```python
from build123d import *

# Parameters (mm, degrees)
SKETCH1_R           = 10
SKETCH1_R_2         = 1.5
SKETCH1_R_3         = 4.5
BOSS_EXTRUDE1_DEPTH = 2
SKETCH1_2_R         = 4.5
BOSS_EXTRUDE2_DEPTH = 4.5
SKETCH2_R           = 1.5
CUT_EXTRUDE1_DEPTH  = 4.5
SKETCH3_R           = 2.75
CUT_EXTRUDE2_DEPTH  = 3.5
CUT_EXTRUDE3_DEPTH  = 3.5
CIRPATTERN1_COUNT   = 25


with BuildPart() as part:
    # Sketch1 → Boss-Extrude1 (new body)
    with BuildSketch(Plane.XY):
        Circle(SKETCH1_R)
        with Locations((0, 7)):
            Circle(SKETCH1_R_2, mode=Mode.SUBTRACT)
        with Locations((7, 0)):
            Circle(SKETCH1_R_2, mode=Mode.SUBTRACT)
        with Locations((0, -7)):
            Circle(SKETCH1_R_2, mode=Mode.SUBTRACT)
        with Locations((-7, 0)):
            Circle(SKETCH1_R_2, mode=Mode.SUBTRACT)
        Circle(SKETCH1_R_3, mode=Mode.SUBTRACT)
    extrude(amount=BOSS_EXTRUDE1_DEPTH)

    # Sketch1_2 → Boss-Extrude2 (add)
    with BuildSketch(Plane.XY):
        Circle(SKETCH1_2_R)
    extrude(amount=BOSS_EXTRUDE2_DEPTH)

    # Sketch2 → Cut-Extrude1 (cut)
    with BuildSketch(Plane(origin=(0, 0, 0), x_dir=(-1, 0, 0), z_dir=(0, 0, -1))):
        Circle(SKETCH2_R)
    extrude(amount=-CUT_EXTRUDE1_DEPTH, mode=Mode.SUBTRACT)

    # Sketch3 → Cut-Extrude2 (cut)
    with BuildSketch(Plane.XY.offset(4.5)):
        Circle(SKETCH3_R)
    extrude(amount=-CUT_EXTRUDE2_DEPTH, mode=Mode.SUBTRACT)

    # Sketch4 → Cut-Extrude3 (cut)
    with BuildSketch(Plane.XY.offset(4.5)):
        with BuildLine():
            Line((-2.976344104, 0.375999701), (-2.728315429, 0.344666392))
            ThreePointArc((-2.728315429, 0.344666392), (-2.70218519, 0.510583192), (-2.665974712, 0.674595311))
            Line((-2.665974712, 0.674595311), (-2.976344104, 0.375999701))
        make_face()
        with BuildLine():
            Line((-2.976344104, 0.375999701), (-2.75, 0))
            ThreePointArc((-2.75, 0), (-2.744573503, 0.172673929), (-2.728315429, 0.344666392))
            Line((-2.728315429, 0.344666392), (-2.976344104, 0.375999701))
        make_face()
    cut_extrude3 = extrude(amount=-CUT_EXTRUDE3_DEPTH, mode=Mode.SUBTRACT)

    # CirPattern1: Cut-Extrude3 ×25 about axis
    cirpattern1_axis = Axis((0, 0, 0), (0, 0, 1))
    for i in range(1, CIRPATTERN1_COUNT):
        add(cut_extrude3.rotate(cirpattern1_axis, i * 360 / CIRPATTERN1_COUNT), mode=Mode.SUBTRACT)


solid = part.part
```
The listing builds one solid part. Answer for the finished solid, in the listing's coordinates (mm). A direction names the side the tool comes from. Round coordinates to 2 decimals unless told otherwise and drop trailing zeros. Write each loop counter-clockwise with the first axis right and the second up, starting at its lowest first coordinate (ties: lowest second). Pieces come first, ordered by that corner, then holes. Notation, with made-up numbers: (58.25, 79) -> (69.25, 79) arc R11 ccw to (69.25, 85) -> close; hole circle Ø1 at (37.25, 86.5). An arc over 180 degrees is marked (long way). Answer as a JSON object with one key per item and string values. Group by question number.
Q1. Determine the mould class of faces 1 (the face through (1, -3, 4.5)), 2 (the face through (-0.59, 4.46, 3.23)), 3 (the face through (-0.325, -8.464, 0.986)) for opening direction X: pulls with the +X half, pulls with the -X half, needs draft (parallel to the pull), parting line crosses it, or undercut.
Q2. Section A-A (z = 0.7) is taken. Write down the section's boundary in (x, y), plus the area to 3 significant figures.
Q3. Section D-D (y = 4) is taken. Write down the section's boundary in (x, z).
Q4. Each of these flat-tipped pins is pushed along its axis until it touches: pin 1 Ø2.5 at (x, y) = (0, 7) entering from +Z; pin 2 Ø3 at (x, y) = (7.5, 3) entering from +Z; pin 3 Ø1 at (y, z) = (4, 3.5) entering from +X; pin 4 Ø2 at (x, z) = (5.5, 1.5) entering from +Y. Where does it stop, or does it pass through?
Q5. Section C-C (y = 7.25) is taken. Write down the section's boundary in (x, z), plus the area to 3 significant figures.
Q6. Straight lines are drawn through the part: line 1 along Y through (x, z) = (0, 0.9); line 2 along Y through (x, z) = (1, 0.4); line 3 along Z through (x, y) = (-7, 2). For each, find the intervals that lie inside material, in ascending order.
Q7. Section B-B (y = -8) is taken. Write down the section's boundary in (x, z).
Q8. Which of the six approach directions +Z, -Z, +X, -X, +Y, -Y give full straight-line access (tool end or side, diameter ignored) to faces 4 (the face through (1.5, 0.07, 0.49)), 5 (the face through (1.3, 1.4, 1))?
Check values:
{
 "1": {"face 1": "needs draft", "face 2": "parting line crosses it", "face 3": "undercut"},
 "2": {"outline": "circle Ø20 at (0, 0); hole circle Ø3 at (-7, 0); hole circle Ø3 at (0, -7); hole circle Ø3 at (0, 0); hole circle Ø3 at (0, 7); hole circle Ø3 at (7, 0)", "area": "279 mm^2"},
 "3": {"outline": "(-9.17, 0) -> (9.17, 0) -> (9.17, 2) -> (2.06, 2) -> (2.06, 4.5) -> (-2.06, 4.5) -> (-2.06, 2) -> (-9.17, 2) -> close"},
 "4": {"pin 1": "through", "pin 2": "z = 2", "pin 3": "x = 2.83", "pin 4": "y = 8.93"},
 "5": {"outline": "(-6.89, 0) -> (-1.48, 0) -> (-1.48, 2) -> (-6.89, 2) -> close; (1.48, 0) -> (6.89, 0) -> (6.89, 2) -> (1.48, 2) -> close", "area": "21.6 mm^2"},
 "6": {"line 1": "-10 to -8.5, -5.5 to -1.5, 1.5 to 5.5, 8.5 to 10", "line 2": "-9.95 to -8.12, -5.88 to -1.12, 1.12 to 5.88, 8.12 to 9.95", "line 3": "0 to 2"},
 "7": {"outline": "(-6, 0) -> (-1.12, 0) -> (-1.12, 2) -> (-6, 2) -> close; (1.12, 0) -> (6, 0) -> (6, 2) -> (1.12, 2) -> close"},
 "8": {"face 4": "+Z, -Z", "face 5": "+Z"}
}
